Geometry check sheet. Reference: the model listing, model coordinates, mm. Give positions to 0.01 mm unless a question says otherwise; leave off trailing zeros. Write each loop counter-clockwise with the first axis right and the second up, starting at its lowest first coordinate (ties: lowest second). Pieces come first, ordered by that corner, then holes. Notation, with made-up numbers: (-36.75, 85.5) - (16.25, 85.5) arc R32 ccw to (16.25, 113.5) - close; hole circle Ø10 at (35.5, 68.25). An arc over 180 degrees is marked (long way). One line per question, with ' | ' between items. Start each with the question number.
Q1. Section check A-A on z = 30. Record the boundary of the cut face in (x, y).
Q2. Gauge pin test, flat end, axial feed: P1, Ø1, axis at y = -0.5, z = 20.5, coming from the -X side. Record the tip position at first contact, or that the pin passes through.
Q3. Thickness scan on L1, parallel to Y at x = -0.1, z = 13.5; L2, parallel to Y at x = 0.4, z = 17. Record the ranges inside material, lowest first. Write a range as [from, to].
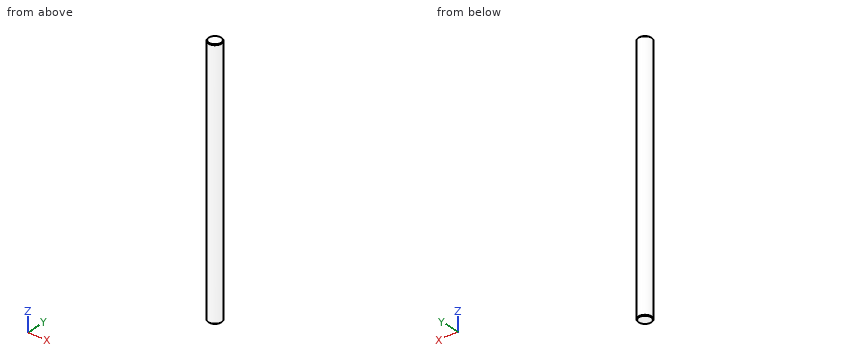
Autodesk Inventor part; units mm, degrees
ref_plane "YZ Plane" through (0, 0, 0) normal (1, 0, 0) x (0, 1, 0)
ref_plane "XZ Plane" through (0, 0, 0) normal (0, 1, 0) x (-1, 0, 0)
ref_plane "XY Plane" through (0, 0, 0) normal (0, 0, 1) x (1, 0, 0)
sketch "スケッチ1" plane through (0, 0, 0) normal (0, 0, 1) x (1, 0, 0)
  circle A0 centre (0, 0) radius 1
  dimension "d0" = 2
extrude "押し出し1" add sketch "スケッチ1" along normal blind 38
chamfer "面取り1" distance 0.09 angle 45 1 edges at (-1, 0, 0)
chamfer "面取り2" distance 0.09 angle 45 1 edges at (-1, 0, 38)
properties part number "motorshaft2x38" material "鋼、合金"
Working result:
1) outline: circle Ø2 at (0, 0)
2) P1: stops at x = -1
3) L1: y = [-0.99, 0.99] | L2: y = [-0.92, 0.92]
